from build123d import *

# Parameters (mm, degrees)
SKETCH1_R                = 8
SKETCH1_R_2              = 3.5
BOSS_EXTRUDE1_DEPTH      = 3
SKETCH2_R                = 8
SKETCH2_R_2              = 5
BOSS_EXTRUDE2_DEPTH      = 6
WRAP3_SECTION_W          = 4
WRAP3_SECTION_H          = 2
WRAP3_ANGLE              = 57.295779513
WRAP3_SECTOR_2_SECTION_W = 4
WRAP3_SECTOR_2_SECTION_H = 2
WRAP3_SECTOR_2_ANGLE     = 57.295779513
CUT_EXTRUDE1_DEPTH       = 4
BOSS_EXTRUDE3_DEPTH      = 9


with BuildPart() as part:
    # Sketch1 → Boss-Extrude1 (new body)
    with BuildSketch(Plane.XY):
        Circle(SKETCH1_R)
        Circle(SKETCH1_R_2, mode=Mode.SUBTRACT)
    extrude(amount=BOSS_EXTRUDE1_DEPTH)

    # Sketch2 → Boss-Extrude2 (add)
    with BuildSketch(Plane.XY.offset(3)):
        Circle(SKETCH2_R)
        Circle(SKETCH2_R_2, mode=Mode.SUBTRACT)
    extrude(amount=BOSS_EXTRUDE2_DEPTH)

    # Wrap3 section (on wrap section) → Wrap3 (revolve, cut)
    with BuildSketch(Plane(origin=(0, 0, 0), x_dir=(-0.8779640629990781, -0.4787265441587198, 0), z_dir=(0.4787265441587198, -0.8779640629990781, 0))):
        with Locations((6, -8)):
            Rectangle(WRAP3_SECTION_W, WRAP3_SECTION_H)
    revolve(axis=Axis((0, 0, 0), (0, 0, -1)), revolution_arc=WRAP3_ANGLE, mode=Mode.SUBTRACT)

    # Wrap3 sector 2 section (on wrap section) → Wrap3 sector 2 (revolve, cut)
    with BuildSketch(Plane(origin=(0, 0, 0), x_dir=(0.8772005042746819, 0.4801242290285337, 0), z_dir=(-0.4801242290285337, 0.8772005042746819, 0))):
        with Locations((6, -8)):
            Rectangle(WRAP3_SECTOR_2_SECTION_W, WRAP3_SECTOR_2_SECTION_H)
    revolve(axis=Axis((0, 0, 0), (0, 0, -1)), revolution_arc=WRAP3_SECTOR_2_ANGLE, mode=Mode.SUBTRACT)

    # Sketch5 → Cut-Extrude1 (cut)
    with BuildSketch(Plane(origin=(0, 0, 0), x_dir=(-1, 0, 0), z_dir=(0, 0, -1))):
        with BuildLine():
            Line((-1.3, 6.776429738), (-1.3, 7.893668349))
            ThreePointArc((-1.3, 7.893668349), (0, -8), (1.3, 7.893668349))
            Line((1.3, 7.893668349), (1.3, 6.776429738))
            ThreePointArc((1.3, 6.776429738), (0, -6.9), (-1.3, 6.776429738))
        make_face()
    extrude(amount=-CUT_EXTRUDE1_DEPTH, mode=Mode.SUBTRACT)

    # Sketch6 → Boss-Extrude3 (add)
    with BuildSketch(Plane(origin=(0, 0, 0), x_dir=(-1, 0, 0), z_dir=(0, 0, -1))):
        with BuildLine():
            Line((-1.3, 7.797149396), (-1.3, 8.576429738))
            Line((-1.3, 8.576429738), (1.3, 8.576429738))
            Line((1.3, 8.576429738), (1.3, 7.797149396))
            ThreePointArc((1.3, 7.797149396), (0, 7.903481047), (-1.3, 7.797149396))
        make_face()
    extrude(amount=-BOSS_EXTRUDE3_DEPTH)


solid = part.part
Read the model definition and answer for the solid it produces. Units are mm, in the model's axes. A direction names the side the tool comes from. Round coordinates to 2 decimals unless told otherwise and drop trailing zeros. Loops run counter-clockwise (first coordinate to the right, second up) from the corner with the lowest first, then second, coordinate; pieces in that order, holes last.
Q1. Determine the mould class of faces 5 (the face through (-0.285, -6.894, 1.972)), 6 (the face through (0, 6, 9)), 7 (the face through (3.233, -1.341, 1.479)) for opening direction X: released by +X, released by -X, zero draft, split by the parting line, or undercut.
Q2. Which of the six approach directions +Z, -Z, +X, -X, +Y, -Y give full straight-line access (tool end or side, diameter ignored) to faces 1 (the face through (2.2, -3.3, 3)), 2 (the face through (1.3, 8, 3)), 3 (the face through (4, -6, 4)), 4 (the face through (5.688, -3.102, 7.986))?
Q3. Consider probe 1 along Y at (x, z) = (0, 1.5); probe 2 along Y at (x, z) = (0, 6.6); probe 3 along X at (y, z) = (-0.5, 0.5). Determine where each line is inside the solid, lowest interval first.
Q4. Each of these flat-tipped pins is pushed along its axis until it touches: pin 1 (3 mm diameter, centred on x = -5.5, y = -1, fed in from +Z); pin 2 (1 mm diameter, centred on x = -5.5, z = 7.5, fed in from -Y) (3 decimals); pin 3 (8 mm diameter, centred on x = 0, y = 0, fed in from +Z); pin 4 (1.5 mm diameter, centred on x = -2, y = 0.5, fed in from -Z). Where does it stop, or does it pass through?
Q5. Section B-B on y = 0 is taken. Write down the section's boundary in (x, z).
Q6. Section A-A on x = 0 is taken. Write down the section's boundary in (y, z).
Q7. Section C-C on z = 6.5 is taken. Write down the section's boundary in (x, y).
Q8. Section D-D on x = -4.75 is taken. Write down the section's boundary in (y, z).
Output:
1. face 5: split by the parting line
1. face 6: zero draft
1. face 7: undercut
2. face 1: +Z
2. face 2: -Z, +X, +Y
2. face 3: -Z
2. face 4: +Z, +X
3. probe 1: y = -6.9 to -3.5, 3.5 to 8.58
3. probe 2: y = -8 to -5, 5 to 8.58
3. probe 3: x = -6.88 to -3.46, 3.46 to 6.88
4. pin 1: stops at z = 7
4. pin 2: stops at y = -6.245
4. pin 3: stops at z = 3
4. pin 4: passes through
5. outline: (-8, 4) - (-6.9, 4) - (-6.9, 0) - (-3.5, 0) - (-3.5, 3) - (-5, 3) - (-5, 7) - (-8, 7) - close; (3.5, 0) - (6.9, 0) - (6.9, 4) - (8, 4) - (8, 7) - (5, 7) - (5, 3) - (3.5, 3) - close
6. outline: (-8, 4) - (-6.9, 4) - (-6.9, 0) - (-3.5, 0) - (-3.5, 3) - (-5, 3) - (-5, 9) - (-8, 9) - close; (3.5, 0) - (8.58, 0) - (8.58, 9) - (5, 9) - (5, 3) - (3.5, 3) - close
7. outline: (-1.3, 7.89) arc R8 ccw (long way) to (1.3, 7.89) - (1.3, 8.58) - (-1.3, 8.58) - close; hole circle Ø10 at (0, 0)
8. outline: (-6.44, 4) - (-5, 4) - (-5, 0) - (5, 0) - (5, 4) - (6.44, 4) - (6.44, 9) - (2.6, 9) - (2.6, 7) - (1.56, 7) - (1.56, 3) - (-1.56, 3) - (-1.56, 7) - (-2.59, 7) - (-2.59, 9) - (-6.44, 9) - close
